Autodesk Inventor part; units mm, degrees
ref_plane "YZ Plane" through (0, 0, 0) normal (1, 0, 0) x (0, 1, 0)
ref_plane "XZ Plane" through (0, 0, 0) normal (0, 1, 0) x (-1, 0, 0)
ref_plane "XY Plane" through (0, 0, 0) normal (0, 0, 1) x (1, 0, 0)
sketch "スケッチ1" plane through (0, 0, 0) normal (0, 0, 1) x (1, 0, 0)
  line L0 (0, 3.1754) -> (2.75, 1.5877)
  line L1 (2.75, 1.5877) -> (2.75, -1.5877)
  line L2 (2.75, -1.5877) -> (0, -3.1754)
  line L3 (0, -3.1754) -> (-2.75, -1.5877)
  line L4 (-2.75, -1.5877) -> (-2.75, 1.5877)
  line L5 (-2.75, 1.5877) -> (0, 3.1754)
  point P0 (0, 0)
  point P1 (0, 0)
  dimension "d0" = 5.5
extrude "押し出し1" add sketch "スケッチ1" along normal blind 35
sketch "スケッチ2" plane through (0, 0, 35) normal (0, 0, 1) x (1, 0, 0)
  circle A0 centre (0, 0) radius 1.5
  dimension "d3" = 3
extrude "押し出し2" add sketch "スケッチ2" along normal blind 6
sketch "スケッチ3" plane through (0, 0, 0) normal (0, 0, -1) x (-1, 0, 0)
  point P0 (0, 0)
hole "穴1" at (0, 0, 0) direction (0, 0, 1) diameter 2.459 depth 8.8 tip angle 118
properties part number "SBD-O3-25" material "真鍮、ソフト イエロー"
Input: part model. Units: mm. Frame: model coordinates. A direction names the side the tool comes from. Give positions to 0.01 mm unless a question says otherwise; leave off trailing zeros. Order: outer loops, then holes, each group sorted by start corner. A loop starts at its lowest first (then second) coordinate and runs counter-clockwise, first axis right, second up. Notation, with made-up numbers: M -36.5,47 L 6.5,47 A14 ccw 6.5,73 Z; hole C -22,40 d11. An arc over 180 degrees is marked long. One line per question, with ' | ' between items.
1) Ray query, L1, parallel to X at y = 0, z = 6.75; L2, parallel to Z at x = 0.55, y = -1.75; L3, parallel to Y at x = 0.4, z = 2.5. Return the intervals inside material, ascending.
Filled in:
L1: x = -2.75 to -1.23, 1.23 to 2.75 | L2: z = 0 to 35 | L3: y = -2.94 to -1.16, 1.16 to 2.94
2) Section A-A on z = 6.5. Output: boundary loops of the cut face in (x, y), and give its area (3 significant figures).
Filled in:
outline: M -2.75,-1.59 L 0,-3.18 L 2.75,-1.59 L 2.75,1.59 L 0,3.18 L -2.75,1.59 Z; hole C 0,0 d2.46 | area: 21.4 mm2
3) Section B-B on z = 15.5. Output: boundary loops of the cut face in (x, y), and give its area (3 significant figures).
Filled in:
outline: M -2.75,-1.59 L 0,-3.18 L 2.75,-1.59 L 2.75,1.59 L 0,3.18 L -2.75,1.59 Z | area: 26.2 mm2
4) Draft query along Y for faces 3 (the face through (0.748, -0.976, 4.462)), 4 (the face through (1.394, -2.37, 17.255)), 5 (the face through (-1.5, -0.07, 37.96)), 6 (the face through (0, 0, 41)). Return one class per face: pulls with the +Y half, pulls with the -Y half, needs draft (parallel to the pull), parting line crosses it, or undercut.
Filled in:
face 3: undercut | face 4: pulls with the -Y half | face 5: parting line crosses it | face 6: needs draft
5) Section C-C on x = 2.3. Output: boundary loops of the cut face in (y, z), and give its area (3 significant figures).
Filled in:
outline: M -1.85,0 L 1.85,0 L 1.85,35 L -1.85,35 Z | area: 129 mm2
6) Access query for faces 1 (the face through (0.064, 0.204, 9.41)), 2 (the face through (-1.3, -1.4, 35)). Directions: +Z, -Z, +X, -X, +Y, -Y. A direction counts if a zero-diameter tool reaches every point of the face in a straight line with its end or side. Return the directions, or none.
Filled in:
face 1: -Z | face 2: +Z
7) Section D-D on z = 38.5. Output: boundary loops of the cut face in (x, y).
Filled in:
outline: C 0,0 d3
